For this review, take the finished solid that the model builds, in its own axes (mm). Face numbers are marked on the shaded views. A direction names the side the tool comes from. Round coordinates to 2 decimals unless told otherwise and drop trailing zeros. Order: outer loops, then holes, each group sorted by start corner. A loop starts at its lowest first (then second) coordinate and runs counter-clockwise, first axis right, second up. Notation, with made-up numbers: (67.25, 76.5) - (71.25, 76.5) arc R8 ccw to (71.25, 88.5) - close; hole circle Ø7 at (3.25, -17). An arc over 180 degrees is marked (long way). One line per question, with ' | ' between items.
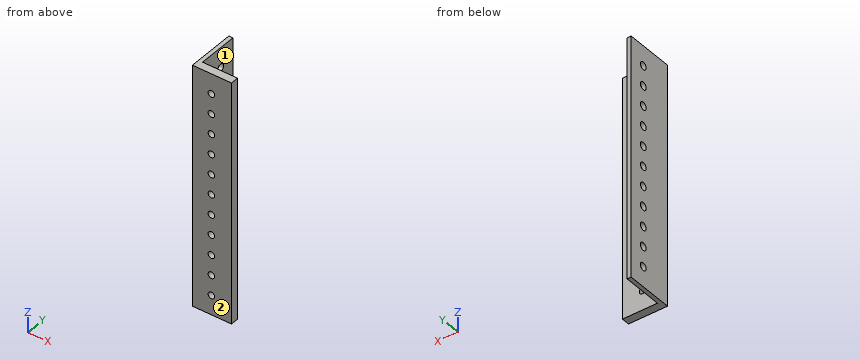
```python
from build123d import *

# Parameters (mm, degrees)
SKETCH1_W           = 152.4
SKETCH1_H           = 30.48
SKETCH1_R           = 2.413
BOSS_EXTRUDE1_DEPTH = 2.54
SKETCH2_W           = 152.4
SKETCH2_H           = 5.08
BOSS_EXTRUDE2_DEPTH = 22.098
SKETCH3_R           = 2.054469346
CUT_EXTRUDE1_DEPTH  = 146.561723888


with BuildPart() as part:
    # Sketch1 → Boss-Extrude1 (new body)
    with BuildSketch(Plane(origin=(0, 0, 0), x_dir=(0, 0, -1), z_dir=(1, 0, 0))):
        with Locations((64.994987224, -0.229680851)):
            Rectangle(SKETCH1_W, SKETCH1_H)
        with Locations((1.494987224, 4.850319149)):
            Circle(SKETCH1_R, mode=Mode.SUBTRACT)
        with Locations((14.194987224, 4.850319149)):
            Circle(SKETCH1_R, mode=Mode.SUBTRACT)
        with Locations((26.894987224, 4.850319149)):
            Circle(SKETCH1_R, mode=Mode.SUBTRACT)
        with Locations((39.594987224, 4.850319149)):
            Circle(SKETCH1_R, mode=Mode.SUBTRACT)
        with Locations((52.294987224, 4.850319149)):
            Circle(SKETCH1_R, mode=Mode.SUBTRACT)
        with Locations((64.994987224, 4.850319149)):
            Circle(SKETCH1_R, mode=Mode.SUBTRACT)
        with Locations((77.694987224, 4.850319149)):
            Circle(SKETCH1_R, mode=Mode.SUBTRACT)
        with Locations((90.394987224, 4.850319149)):
            Circle(SKETCH1_R, mode=Mode.SUBTRACT)
        with Locations((103.094987224, 4.850319149)):
            Circle(SKETCH1_R, mode=Mode.SUBTRACT)
        with Locations((115.794987224, 4.850319149)):
            Circle(SKETCH1_R, mode=Mode.SUBTRACT)
        with Locations((128.494987224, 4.850319149)):
            Circle(SKETCH1_R, mode=Mode.SUBTRACT)
    extrude(amount=BOSS_EXTRUDE1_DEPTH)

    # Sketch2 → Boss-Extrude2 (add)
    with BuildSketch(Plane(origin=(2.54, 0, 0), x_dir=(0, 0, -1), z_dir=(1, 0, 0))):
        with Locations((64.994987224, -12.929680851)):
            Rectangle(SKETCH2_W, SKETCH2_H)
    extrude(amount=BOSS_EXTRUDE2_DEPTH)

    # Sketch3 → Cut-Extrude1 (cut, through all)
    with BuildSketch(Plane(origin=(0, -10.389680851, 0), x_dir=(1, 0, 0), z_dir=(0, 1, 0))):
        with Locations(Location((11.938, 1.494987224, 0), (0, 0, 270))):
            Circle(SKETCH3_R)
        with Locations(Location((11.938, 14.236129272, 0), (0, 0, 270))):
            Circle(SKETCH3_R)
        with Locations(Location((11.938, 26.977271321, 0), (0, 0, 270))):
            Circle(SKETCH3_R)
        with Locations(Location((11.938, 39.71841337, 0), (0, 0, 270))):
            Circle(SKETCH3_R)
        with Locations(Location((11.938, 52.459555419, 0), (0, 0, 270))):
            Circle(SKETCH3_R)
        with Locations(Location((11.938, 65.200697467, 0), (0, 0, 270))):
            Circle(SKETCH3_R)
        with Locations(Location((11.938, 77.941839516, 0), (0, 0, 270))):
            Circle(SKETCH3_R)
        with Locations(Location((11.938, 90.682981565, 0), (0, 0, 270))):
            Circle(SKETCH3_R)
        with Locations(Location((11.938, 103.424123614, 0), (0, 0, 270))):
            Circle(SKETCH3_R)
        with Locations(Location((11.938, 116.165265662, 0), (0, 0, 270))):
            Circle(SKETCH3_R)
        with Locations(Location((11.938, 128.906407711, 0), (0, 0, 270))):
            Circle(SKETCH3_R)
    extrude(amount=-CUT_EXTRUDE1_DEPTH, mode=Mode.SUBTRACT)


solid = part.part
```
(1) We need section A-A on z = -90. State the section outline as (x, y) points, plus the area to 3 significant figures.
Output values:
outline: (0, -15.47) - (10, -15.47) - (10, -10.39) - (2.54, -10.39) - (2.54, 2.47) - (0, 2.47) - close; (0, 7.23) - (2.54, 7.23) - (2.54, 15.01) - (0, 15.01) - close; (13.88, -15.47) - (24.64, -15.47) - (24.64, -10.39) - (13.88, -10.39) - close | area: 158 mm^2
(2) We need section D-D on z = -9.5. State the section outline as (x, y) points.
Output values:
outline: (0, -15.47) - (24.64, -15.47) - (24.64, -10.39) - (2.54, -10.39) - (2.54, 15.01) - (0, 15.01) - close
(3) We need section B-B on y = -12. Give the number of separate pieces and of enclosed holes in the cut face, plus the area to 3 significant figures.
Output values:
separate pieces: 1 | enclosed holes: 11 | area: 3,610 mm^2
(4) Insertion check: pin 1 (6.5 mm diameter, centred on y = 4.85, z = -1.49, fed in from +X); pin 2 (12 mm diameter, centred on x = 21.5, z = -55.5, fed in from +Y). Each pin has a flat end and moves straight along its axis. Give the tip position at first contact, or say it passes through.
Output values:
pin 1: x = 2.54 | pin 2: y = -10.39
(5) We need section C-C on x = 20.25. State the section outline as (y, z) points, plus the area to 3 significant figures.
Output values:
outline: (-15.47, -141.19) - (-10.39, -141.19) - (-10.39, 11.21) - (-15.47, 11.21) - close | area: 774 mm^2
(6) For probe 1 along X at (y, z) = (-5.5, -80.5); probe 2 along Y at (x, z) = (14.75, -9); probe 3 along Y at (x, z) = (1, 0), list the stretches that pass through material, from the lowest coordinate up. Write a range as [from, to].
Output values:
probe 1: [0, 2.54] | probe 2: [-15.47, -10.39] | probe 3: [-15.47, 2.96], [6.74, 15.01]
(7) For the marked faces 1 and 2, list the 3-axis set-ups (+Z, -Z, +X, -X, +Y, -Y) from which the entire face can be reached by the end or side of a thin tool; tool diameter is ignored.
Output values:
face 1: +Z, -Z, +X, +Y | face 2: +Z, -Z, +X, -X, -Y
